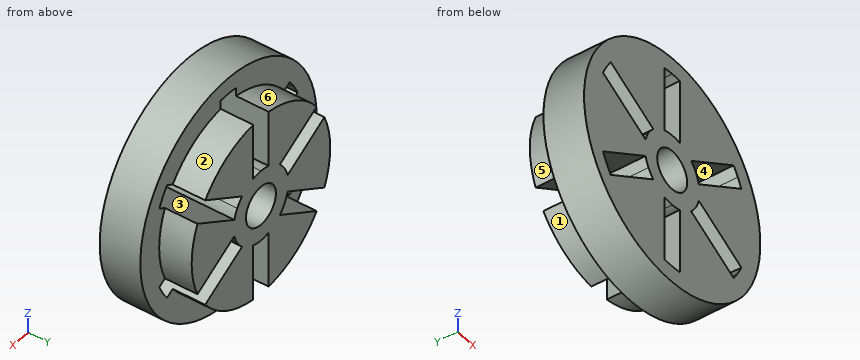
```python
from build123d import *

# Parameters (mm, degrees)
SKETCH1_R           = 28.5
BOSS_EXTRUDE1_DEPTH = 10
SKETCH2_R           = 22.4
BOSS_EXTRUDE2_DEPTH = 8
SKETCH3_R           = 4.85
CUT_EXTRUDE1_DEPTH  = 45.141816909
CUT_EXTRUDE2_DEPTH  = 45.141816909
CIRPATTERN1_COUNT   = 6


with BuildPart() as part:
    # Sketch1 → Boss-Extrude1 (new body)
    with BuildSketch(Plane(origin=(0, 0, 0), x_dir=(1, 0, 0), z_dir=(0, 1, 0))):
        with Locations(Location((0, 0, 0), (0, 0, 270))):
            Circle(SKETCH1_R)
    extrude(amount=BOSS_EXTRUDE1_DEPTH)

    # Sketch2 → Boss-Extrude2 (add)
    with BuildSketch(Plane(origin=(0, 10, 0), x_dir=(1, 0, 0), z_dir=(0, 1, 0))):
        with Locations(Location((0, 0, 0), (0, 0, 270))):
            Circle(SKETCH2_R)
    extrude(amount=BOSS_EXTRUDE2_DEPTH)

    # Sketch3 → Cut-Extrude1 (cut, through all)
    with BuildSketch(Plane(origin=(0, 18, 0), x_dir=(1, 0, 0), z_dir=(0, 1, 0))):
        with Locations(Location((0, 0, 0), (0, 0, 270))):
            Circle(SKETCH3_R)
    extrude(amount=-CUT_EXTRUDE1_DEPTH, mode=Mode.SUBTRACT)

    # Sketch9 → Cut-Extrude2 (cut, through all)
    with BuildSketch(Plane.XZ):
        with BuildLine():
            Line((0, 24.5), (0, 8.85))
            ThreePointArc((0, 8.85), (1.260616548, 8.759757184), (2.495524262, 8.490869134))
            Line((2.495524262, 8.490869134), (2.495524262, 24.372573903))
            ThreePointArc((2.495524262, 24.372573903), (1.249387725, 24.468122738), (0, 24.5))
        make_face()
        with BuildLine():
            ThreePointArc((-2.5, 8.489552403), (-1.26292542, 8.759424603), (0, 8.85))
            Line((0, 8.85), (0, 24.5))
            ThreePointArc((0, 24.5), (-1.251634383, 24.468007916), (-2.5, 24.372115214))
            Line((-2.5, 24.372115214), (-2.5, 8.489552403))
        make_face()
    cut_extrude2 = extrude(amount=-CUT_EXTRUDE2_DEPTH, mode=Mode.SUBTRACT)

    # CirPattern1: Cut-Extrude2 ×6 about axis
    cirpattern1_axis = Axis((0, 0, 0), (0, 1, 0))
    for i in range(1, CIRPATTERN1_COUNT):
        add(cut_extrude2.rotate(cirpattern1_axis, i * 360 / CIRPATTERN1_COUNT), mode=Mode.SUBTRACT)


solid = part.part
```
Verification items for the finished model (mm, model axes). Face numbers are marked on the shaded views. A direction names the side the tool comes from. Round coordinates to 2 decimals unless told otherwise and drop trailing zeros. Write each loop counter-clockwise with the first axis right and the second up, starting at its lowest first coordinate (ties: lowest second). Pieces come first, ordered by that corner, then holes.
1. Access from +Z, -Z, +X, -X, +Y, -Y to the whole of each face (thin tool, end or side, straight path). Record for the marked faces 1, 2 and 3.
2. Draft check along Z on the marked faces 4, 5 and 6. Enter one of: +Z half, -Z half, draft (parallel to the pull), parting line (faces both ways), or undercut.
3. Gauge pin test, flat ends, axial feed: P1, Ø8, axis at y = 5, z = 18.5, coming from the +X side; P2, Ø4, axis at x = -14.5, z = -8.5, coming from the -Y side; P3, Ø11, axis at x = 0, z = 0, coming from the +Y side; P4, Ø1, axis at y = 4, z = 6.5, coming from the +X side. Record the tip position at first contact, or that the pin passes through.
4. Section check A-A on z = 0. Enter the section's corners in (x, y).
5. Section check B-B on x = -7. Enter the section's corners in (y, z), plus the area to 3 significant figures.
6. Section check D-D on y = 7. State how many separate pieces and enclosed holes the cut face has, plus the area to 3 significant figures.
7. Scan lines: L1, parallel to X at y = 9, z = 0; L2, parallel to X at y = 12.75, z = 0; L3, parallel to Z at x = 12, y = 16.5. Record each from-to range of solid material in increasing order.
8. Section check C-C on y = 12.25. Enter the section's corners in (x, z) (3 decimals).
Answer:
1. face 1: -Z, -X, +Y
1. face 2: +Z, +X, +Y
1. face 3: +Y, -Y
2. face 4: undercut
2. face 5: parting line
2. face 6: +Z half
3. P1: stops at x = 24.54
3. P2: passes through
3. P3: stops at y = 18
3. P4: stops at x = 27.86
4. outline: (-28.5, 0) - (-4.85, 0) - (-4.85, 18) - (-22.4, 18) - (-22.4, 10) - (-28.5, 10) - close; (4.85, 0) - (28.5, 0) - (28.5, 10) - (22.4, 10) - (22.4, 18) - (4.85, 18) - close
5. outline: (0, -27.63) - (10, -27.63) - (10, -21.28) - (18, -21.28) - (18, -6.93) - (0, -6.93) - close; (0, -5.42) - (18, -5.42) - (18, 5.42) - (0, 5.42) - close; (0, 6.92) - (18, 6.92) - (18, 21.28) - (10, 21.28) - (10, 27.63) - (0, 27.63) - close
5. area: 839 mm2
6. separate pieces: 1
6. enclosed holes: 7
6. area: 2,010 mm2
7. L1: x = -28.5 to -4.85, 4.85 to 28.5
7. L2: x = -22.4 to -4.85, 4.85 to 22.4
7. L3: z = -18.91 to -9.81, -4.04 to 4.05, 9.81 to 18.91
8. outline: (-20.528, 8.965) arc R22.4 ccw to (-20.526, -8.969) - (-8.601, -2.084) arc R8.85 ccw to (-6.102, -6.41) - (-18.028, -13.295) arc R22.4 ccw to (-2.496, -22.261) - (-2.496, -8.491) arc R8.85 ccw to (2.5, -8.49) - (2.5, -22.26) arc R22.4 ccw to (18.03, -13.291) - (6.106, -6.407) arc R8.85 ccw to (8.602, -2.08) - (20.528, -8.965) arc R22.4 ccw to (20.526, 8.969) - (8.601, 2.084) arc R8.85 ccw to (6.102, 6.41) - (18.028, 13.295) arc R22.4 ccw to (2.496, 22.261) - (2.496, 8.491) arc R8.85 ccw to (-2.5, 8.49) - (-2.5, 22.26) arc R22.4 ccw to (-18.03, 13.291) - (-6.106, 6.407) arc R8.85 ccw to (-8.602, 2.08) - close; hole circle Ø9.7 at (0, 0)
